from build123d import *

# Parameters (mm, degrees)
F0_R          = 24.13
F0_R_2        = 20.447
F1_DEPTH      = 1130.3
F3_DEPTH      = 24.131
F3_DEPTH_BACK = 24.131
F5_DEPTH      = 24.131
F5_DEPTH_BACK = 24.131
F8_W          = 178.4191885963
F8_H          = 167.3920117319
F9_DEPTH      = 50.8
F9_DEPTH_BACK = 20.32


with BuildPart() as f1:
    # F0 (on Top) → F1 (new body)
    with BuildSketch(Plane.XY):
        Circle(F0_R)
        Circle(F0_R_2, mode=Mode.SUBTRACT)
    extrude(amount=F1_DEPTH)

    # F2 (on Right) → F3 (cut, two sides)
    with BuildSketch(Plane.YZ) as f3_sk:
        Polygon((24.13, 1089.8050517994), (24.13, 1130.3), (-24.13, 1130.3), align=None)
    extrude(amount=-F3_DEPTH, mode=Mode.SUBTRACT)
    extrude(f3_sk.sketch, amount=F3_DEPTH_BACK, mode=Mode.SUBTRACT)

    # F4 (on Front) → F5 (cut, two sides)
    with BuildSketch(Plane.XZ) as f5_sk:
        Polygon((-28.575, 0), (28.575, 0), (-28.575, 29.0972948719), align=None)
    extrude(amount=F5_DEPTH, mode=Mode.SUBTRACT)
    extrude(f5_sk.sketch, amount=-F5_DEPTH_BACK, mode=Mode.SUBTRACT)

    # F8 (on line) → F9 (cut, two sides)
    with BuildSketch(Plane(origin=(2.9412132624, -6.4824828952, 5.7768372862), x_dir=(-0.9471380058, -0.2395200516, 0.2134472836), z_dir=(-0.3208264297, 0.7071067812, -0.6301352252))) as f9_sk:
        with Locations((5.3417463787, 7.3568988591)):
            Rectangle(F8_W, F8_H)
    extrude(amount=F9_DEPTH, mode=Mode.SUBTRACT)
    extrude(f9_sk.sketch, amount=-F9_DEPTH_BACK, mode=Mode.SUBTRACT)


solid = f1.part
Check sheet for the modelled part. Datum: model origin and axes. Units: mm. Coordinates: 2 decimals unless noted, no trailing zeros. Loops run counter-clockwise (first coordinate to the right, second up) from the corner with the lowest first, then second, coordinate; pieces in that order, holes last. Notation, with made-up numbers: (37.25, 76) -> (96.25, 76) arc R20 cw to (96.25, 83) -> close; hole circle Ø1 at (-3, -20). An arc over 180 degrees is marked (long way). Answer in a Markdown table with one row per item.
1. Release check for a two-part mould opening along Y. For faces 1 (the face through (-16.226, -12.442, 566.247)), 2 (the face through (17.99, 10.2, 49.08)), 3 (the face through (11.13, -21.41, 565.39)) record: released by +Y, released by -Y, zero draft, split by the parting line, or undercut.
Check values:
| item | result |
|---|---|
| face 1 | undercut |
| face 2 | released by +Y |
| face 3 | split by the parting line |
2. Sectioned sample at C-C, the plane z = 695. Record the boundary of the cut face in (x, y).
Check values:
| item | result |
|---|---|
| outline | circle Ø48.26 at (0, 0); hole circle Ø40.89 at (0, 0) |
3. Sectioned sample at A-A, the plane x = 9.5. Record the boundary of the cut face in (y, z).
Check values:
| item | result |
|---|---|
| outline | (-22.18, 17.07) -> (-18.11, 21.64) -> (-18.11, 1125.25) -> (-22.18, 1128.66) -> close; (18.11, 62.28) -> (22.18, 66.85) -> (22.18, 1091.44) -> (18.11, 1094.86) -> close |
4. Material ranges on line 1 along X through (y, z) = (0, 696.5); line 2 along X through (y, z) = (-2.5, 974), recorded low to high. Write a range as [from, to].
Check values:
| item | result |
|---|---|
| line 1 | x = [-24.13, -20.45], [20.45, 24.13] |
| line 2 | x = [-24, -20.29], [20.29, 24] |
5. Sectioned sample at B-B, the plane y = 0. Record the boundary of the cut face in (x, z).
Check values:
| item | result |
|---|---|
| outline | (-24.13, 59.08) -> (-20.45, 57.21) -> (-20.45, 1110.05) -> (-24.13, 1110.05) -> close; (20.45, 36.39) -> (24.13, 34.51) -> (24.13, 1110.05) -> (20.45, 1110.05) -> close |
6. Go/stop test with flat-tipped pins: pin 1 (6 mm diameter, centred on y = -5.5, z = 450, fed in from -X); pin 2 (4 mm diameter, centred on x = 7.5, z = 505.5, fed in from +Y); pin 3 (6 mm diameter, centred on x = 7.5, z = 958.5, fed in from +Y); pin 4 (10 mm diameter, centred on x = -3.5, y = -11.5, fed in from -Z). Record where each tip stops, or that it passes through.
Check values:
| item | result |
|---|---|
| pin 1 | stops at x = -24 |
| pin 2 | stops at y = 23.49 |
| pin 3 | stops at y = 23.71 |
| pin 4 | passes through |
